Could you check a few things on this model? Use its own coordinates, in mm. A direction names the side the tool comes from. Round coordinates to 2 decimals unless told otherwise and drop trailing zeros. Order: outer loops, then holes, each group sorted by start corner. A loop starts at its lowest first (then second) coordinate and runs counter-clockwise, first axis right, second up. Notation, with made-up numbers: M 57.5,2.25 L 76.5,2.25 A32 ccw 76.5,37.25 Z; hole C 25.25,76.5 d4. An arc over 180 degrees is marked long. Write each question's results on one line, items separated by ' | '. Start each with the question number.
1. Suppose I cut it at A-A on z = 3.25. Give the number of separate pieces and of enclosed holes in the cut face, and give its area (3 significant figures).
2. I'm going to push flat-ended pins straight in: pin 1 (1.5 mm diameter, centred on x = 35.5, z = 3, fed in from +Y); pin 2 (1.2 mm diameter, centred on x = 77.5, z = 4.5, fed in from +Y) (3 decimals); pin 3 (2 mm diameter, centred on y = 3, z = 4, fed in from -X) (3 decimals); pin 4 (1.2 mm diameter, centred on y = 78, z = 3.5, fed in from +X) (3 decimals). Where does each tip first touch, or does it pass through?
3. Please list where these lines run through material, in increasing order: L1, parallel to Y at x = 77, z = 2.7 (3 decimals); L2, parallel to Z at x = 8.5, y = 57.5.
4. We'd pull the mould along X, two halves only. Please class faces 1 (the flat face through (22.575, 79, 4)), 2 (the flat face through (79, 58.675, 4)), 3 (the flat face through (81.25, 40, 2)): released by +X, released by -X, zero draft, split by the parting line, or undercut.
5. Suppose I cut it at B-B on x = 48.5. Write out the boundary of the cut face in (y, z).
6. For faces 4 (the flat face through (79, 60.675, 4)), 5 (the flat face through (5, 60, 4)), 6 (the flat face through (20.575, 2, 4)), 7 (the flat face through (79, 22.575, 4)), which set-ups out of +Z, -Z, +X, -X, +Y, -Y let a thin tool reach every point of the face, with its end or its side?
from build123d import *

# Parameters (mm, degrees)
SKETCH_W      = 81.25
SKETCH_H      = 81.25
PAD_DEPTH     = 2
FILLET_R      = 5.05
SKETCH001_W   = 2
SKETCH001_H   = 5
SKETCH001_W_2 = 5
SKETCH001_H_2 = 2
PAD001_DEPTH  = 4


with BuildPart() as part:
    # Sketch → Pad (new body)
    with BuildSketch(Plane.XY):
        with Locations((40.625, 40.625)):
            Rectangle(SKETCH_W, SKETCH_H)
    extrude(amount=PAD_DEPTH)

    # Fillet
    fillet_edges = [part.edges().sort_by_distance(p)[0] for p in [
        (81.25, 0, 1),
        (0, 0, 1),
        (0, 81.25, 1),
        (81.25, 81.25, 1),
    ]]
    fillet(fillet_edges, radius=FILLET_R)

    # Sketch001 (on Face5 of Fillet) → Pad001 (join)
    with BuildSketch(Plane.XY.offset(2)):
        with Locations((21.575, 78.75)):
            Rectangle(SKETCH001_W, SKETCH001_H)
        with Locations((40.625, 78.75)):
            Rectangle(SKETCH001_W, SKETCH001_H)
        with Locations((59.675, 78.75)):
            Rectangle(SKETCH001_W, SKETCH001_H)
        with Locations((40.625, 2.5)):
            Rectangle(SKETCH001_W, SKETCH001_H)
        with Locations((59.675, 2.5)):
            Rectangle(SKETCH001_W, SKETCH001_H)
        with Locations((21.575, 2.5)):
            Rectangle(SKETCH001_W, SKETCH001_H)
        with Locations((78.75, 40.625)):
            Rectangle(SKETCH001_W_2, SKETCH001_H_2)
        with Locations((2.5, 40.625)):
            Rectangle(SKETCH001_W_2, SKETCH001_H_2)
        with Locations((78.75, 59.675)):
            Rectangle(SKETCH001_W_2, SKETCH001_H_2)
        with Locations((78.75, 21.575)):
            Rectangle(SKETCH001_W_2, SKETCH001_H_2)
        with Locations((2.5, 59.675)):
            Rectangle(SKETCH001_W_2, SKETCH001_H_2)
        with Locations((2.5, 21.575)):
            Rectangle(SKETCH001_W_2, SKETCH001_H_2)
    extrude(amount=PAD001_DEPTH)


solid = part.part
Filled sheet:
1) separate pieces: 12 | enclosed holes: 0 | area: 120 mm^2
2) pin 1: passes through | pin 2: stops at y = 60.675 | pin 3: stops at x = 20.575 | pin 4: stops at x = 60.675
3) L1: y = 20.575 to 22.575, 39.625 to 41.625, 58.675 to 60.675 | L2: z = 0 to 2
4) face 1: undercut | face 2: zero draft | face 3: released by +X
5) outline: M 0,0 L 81.25,0 L 81.25,2 L 0,2 Z
6) face 4: +Z, +X, -X, +Y | face 5: +Z, +Y, -Y | face 6: +Z, -X, +Y, -Y | face 7: +Z, +X, -X
